Verification items for this drawing (mm, ordinates from the low corner). A direction names the side the tool comes from. Round coordinates to 2 decimals unless told otherwise and drop trailing zeros. Loops run counter-clockwise (first coordinate to the right, second up) from the corner with the lowest first, then second, coordinate; pieces in that order, holes last. Notation, with made-up numbers: M 13.25,81.5 L 60.25,81.5 A26 cw 60.25,116.5 Z; hole C -17.75,18 d3. An arc over 180 degrees is marked long. Use one line per item in the form item = value. Start each with the question number.
1. Cross-section at D-D (y = 5). Record the boundary of the cut face in (x, z), then the cut area to 3 significant figures.
2. Cross-section at A-A (y = 16.5). Record the boundary of the cut face in (x, z), then the cut area to 3 significant figures.
3. Draft check along Y on the marked faces 3, 4, 5 and 6. Enter one of: pulls with the +Y half, pulls with the -Y half, needs draft (parallel to the pull), parting line crosses it, or undercut.
4. Cross-section at B-B (z = 2). Record the boundary of the cut face in (x, y).
5. Go/stop test with a flat-tipped pin: pin 1 (2 mm diameter, centred on y = 15, z = 1, fed in from +X). Record where the tip stops, or that it passes through.
6. Set-up check for the marked faces 1 and 2: record each of +Z, -Z, +X, -X, +Y, -Y from which the full face is reachable in a straight line by a thin tool's end or side.
7. Material ranges on line 1 (Y direction, x = 2.5, z = 2.65); line 2 (Y direction, x = 1.5, z = 1.85); line 3 (X direction, y = 18.5, z = 1.5), recorded low to high.
8. Cross-section at C-C (x = 2.5). Record the boundary of the cut face in (y, z).
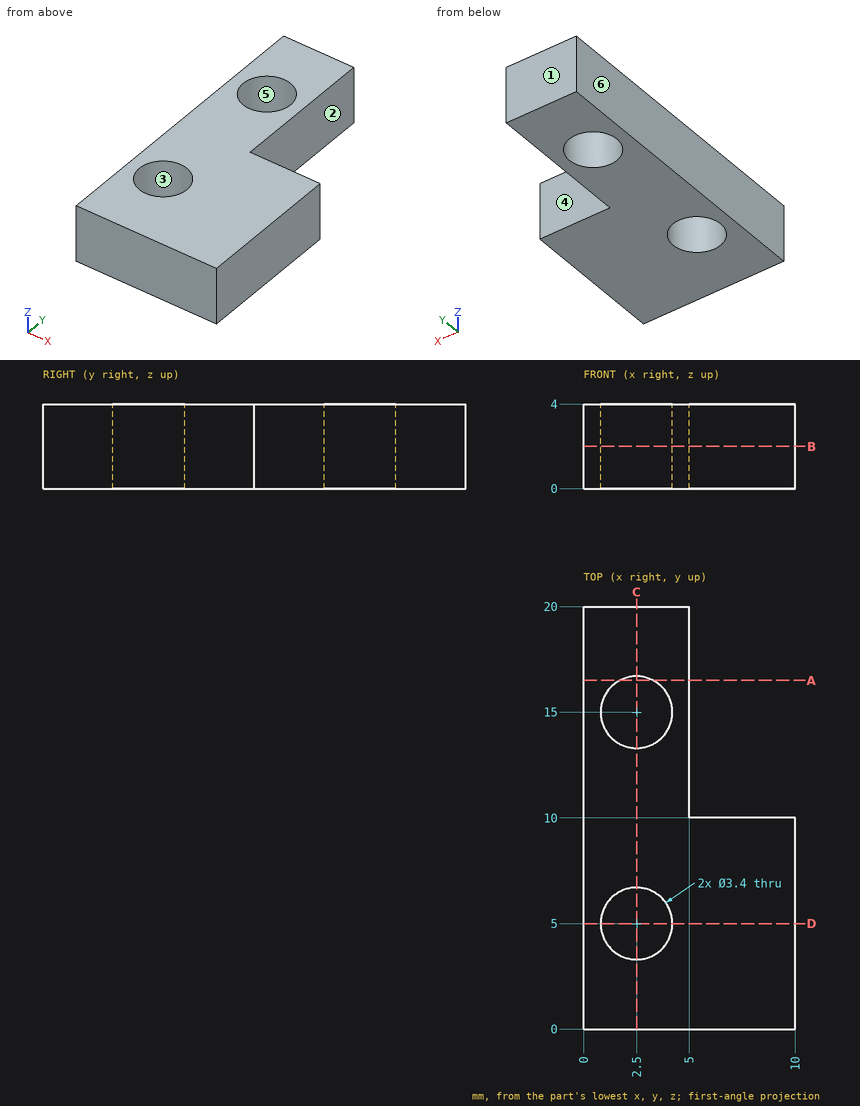
Reported:
q1.outline = M 0,0 L 0.8,0 L 0.8,4 L 0,4 Z; M 4.2,0 L 10,0 L 10,4 L 4.2,4 Z
q1.area = 26.4 mm²
q2.outline = M 0,0 L 1.7,0 L 1.7,4 L 0,4 Z; M 3.3,0 L 5,0 L 5,4 L 3.3,4 Z
q2.area = 13.6 mm²
q3.face_3 = undercut
q3.face_4 = pulls with the +Y half
q3.face_5 = undercut
q3.face_6 = needs draft
q4.outline = M 0,0 L 10,0 L 10,10 L 5,10 L 5,20 L 0,20 Z; hole C 2.5,5 d3.4; hole C 2.5,15 d3.4
q5.pin_1 = 5
q6.face_1 = +Z, -Z, +X, -X, +Y
q6.face_2 = +Z, -Z, +X, +Y
q7.line_1 = 0 to 3.3, 6.7 to 13.3, 16.7 to 20
q7.line_2 = 0 to 3.63, 6.37 to 13.63, 16.37 to 20
q7.line_3 = 0 to 5
q8.outline = M 0,0 L 3.3,0 L 3.3,4 L 0,4 Z; M 6.7,0 L 13.3,0 L 13.3,4 L 6.7,4 Z; M 16.7,0 L 20,0 L 20,4 L 16.7,4 Z
